The drawing under review shows one solid part. Ordinate dimensions are in mm from its lowest x, y, z. A direction names the side the tool comes from. Give positions to 0.01 mm unless a question says otherwise; leave off trailing zeros. Write each loop counter-clockwise with the first axis right and the second up, starting at its lowest first coordinate (ties: lowest second). Pieces come first, ordered by that corner, then holes. Notation, with made-up numbers: M 20,68.5 L 63,68.5 A22 cw 63,91.5 Z; hole C -32.5,17 d4. An arc over 180 degrees is marked long. Answer as a JSON object with one key per item and string values. Group by question number.
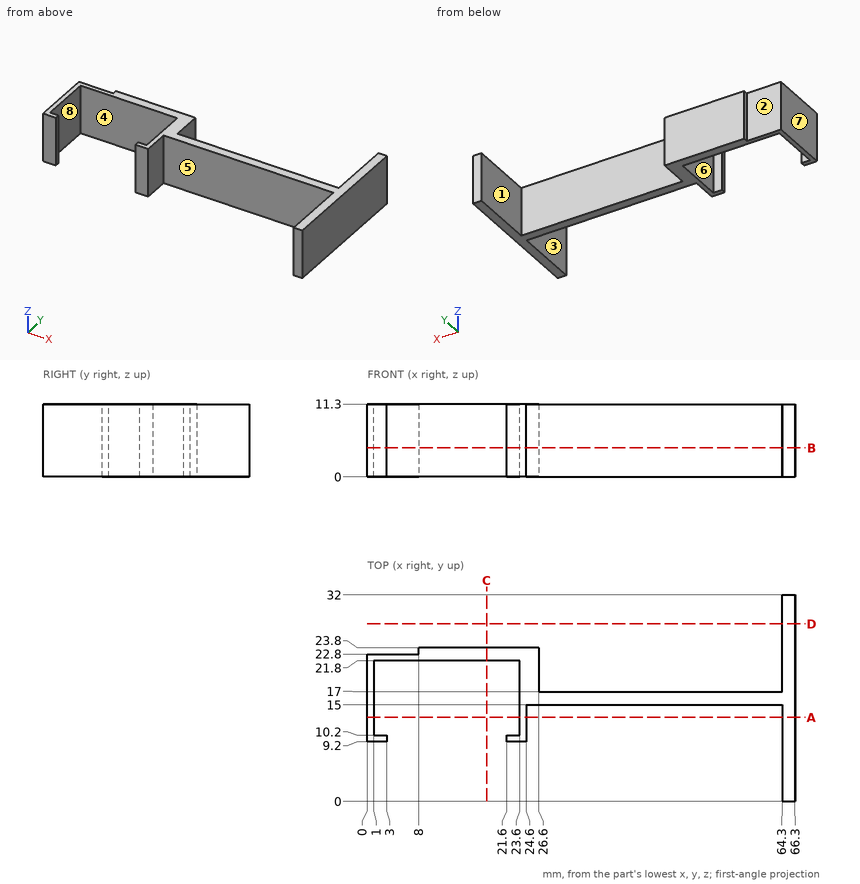
Item 1: Consider section D-D (y = 27.5). Give the boundary of the cut face in (x, z).
Item 2: Insertion check: P1, Ø3.5, axis at x = 17.5, z = 3.5, coming from the +Y side; P2, Ø3.5, axis at x = 24, z = 3, coming from the -Y side; P3, Ø4, axis at y = 5, z = 6.5, coming from the -X side. Each pin has a flat end and moves straight along its axis. Give the tip position at first contact, or say it passes through.
Item 3: Machinability: for the marked faces 1, 2, 3 and 4, which of the approach directions +Z, -Z, +X, -X, +Y, -Y give a long, thin tool a straight path to every point of the face, cutting with its end or side? Answer none if there is none.
Item 4: Draft analysis for pull direction Y (two halves, no side actions). For the marked faces 5, 6, 7 and 8, state which applies: released by +Y, released by -Y, zero draft, split by the parting line, or undercut.
Item 5: To check wall thickness, follow probe 1 along X at (y, z) = (19.5, 7.25); probe 2 along X at (y, z) = (16, 7.25); probe 3 along X at (y, z) = (22, 8.5). State the ranges of each line that lie inside material, in increasing order.
Item 6: Consider section C-C (x = 18.5). Give the boundary of the cut face in (y, z).
Item 7: Consider section B-B (z = 4.5). Give the boundary of the cut face in (x, y), plus the area to 3 significant figures.
Item 8: Consider section A-A (y = 13). Give the boundary of the cut face in (x, z), plus the area to 3 significant figures.
Result set:
{
 "1": {"outline": "M 64.3,0 L 66.3,0 L 66.3,11.3 L 64.3,11.3 Z"},
 "2": {"P1": "stops at y = 23.8", "P2": "stops at y = 9.2", "P3": "stops at x = 64.3"},
 "3": {"face 1": "+Z, -Z, +Y", "face 2": "+Z, -Z, -X, +Y", "face 3": "+Z, -Z, -Y", "face 4": "+Z, -Z"},
 "4": {"face 5": "released by -Y", "face 6": "undercut", "face 7": "zero draft", "face 8": "undercut"},
 "5": {"probe 1": "x = 0 to 1, 23.6 to 26.6, 64.3 to 66.3", "probe 2": "x = 0 to 1, 23.6 to 66.3", "probe 3": "x = 0 to 26.6, 64.3 to 66.3"},
 "6": {"outline": "M 21.8,0 L 23.8,0 L 23.8,11.3 L 21.8,11.3 Z"},
 "7": {"outline": "M 0,9.2 L 3,9.2 L 3,10.2 L 1,10.2 L 1,21.8 L 23.6,21.8 L 23.6,10.2 L 21.6,10.2 L 21.6,9.2 L 24.6,9.2 L 24.6,15 L 64.3,15 L 64.3,0 L 66.3,0 L 66.3,32 L 64.3,32 L 64.3,17 L 26.6,17 L 26.6,23.8 L 8,23.8 L 8,22.8 L 0,22.8 Z", "area": "227 mm^2"},
 "8": {"outline": "M 0,0 L 1,0 L 1,11.3 L 0,11.3 Z; M 23.6,0 L 24.6,0 L 24.6,11.3 L 23.6,11.3 Z; M 64.3,0 L 66.3,0 L 66.3,11.3 L 64.3,11.3 Z", "area": "45.2 mm^2"}
}
